Could you check a few things on this model? Use its own coordinates, in mm. Coordinates: 2 decimals unless noted, no trailing zeros. Write each loop counter-clockwise with the first axis right and the second up, starting at its lowest first coordinate (ties: lowest second). Pieces come first, ordered by that corner, then holes. Notation, with made-up numbers: M 25,80.25 L 60,80.25 A26 ccw 60,99.25 Z; hole C -10,22 d2. An arc over 180 degrees is marked long. Answer as CSV lines item,"result". Start each with the question number.
Item 1: I'm going to push flat-ended pins straight in: P1, Ø8, axis at x = -7.5, y = 6.5, coming from the +Z side; P2, Ø3, axis at y = 6, z = 58, coming from the +X side; P3, Ø6, axis at x = -14.5, z = 56.5, coming from the +Y side. Where does each tip first touch, or does it pass through?
Item 2: Suppose I cut it at A-A, the plane z = 27. Write out the boundary of the cut face in (x, y).
Item 3: Suppose I cut it at B-B, the plane y = 15.75. Write out the boundary of the cut face in (x, z).
Item 4: If I drill on line 1 along Y through (x, z) = (-3, 68); line 2 along X through (y, z) = (11.5, 32); line 3 along Y through (x, z) = (-14.75, 41), over which ranges is the centre line in solid material (lowest first)? Write a range as [from, to].
```python
from build123d import *

# Parameters (mm, degrees)
SALIENTE_EXTRUIR1_DEPTH = 77
CORTAR_EXTRUIR1_REACH   = 15.696
CROQUIS2_R              = 1.6


with BuildPart() as part:
    # Croquis1 → Saliente-Extruir1 (new body)
    with BuildSketch(Plane.XY):
        Polygon((-22, 0), (-17.180905327, 0), (0, 13.666629237), (0, 17.5), align=None)
    extrude(amount=SALIENTE_EXTRUIR1_DEPTH)

    # Croquis2 → Cortar-Extruir1 (cut, up to next)
    with BuildSketch(Plane(origin=(-8.52578298, 10.718127175, 0), x_dir=(0.782601054, 0.622523566, 0), z_dir=(-0.622523566, 0.782601054, 0)), mode=Mode.PRIVATE) as cortar_extruir1_sk1:
        with Locations((1.507798766, -5)):
            Circle(CROQUIS2_R)
    cortar_extruir1_tool1 = extrude(cortar_extruir1_sk1.sketch, amount=-CORTAR_EXTRUIR1_REACH, mode=Mode.PRIVATE) & part.part
    add(cortar_extruir1_tool1.solids().sort_by_distance((-7.345778, 11.656767, 5))[0], mode=Mode.SUBTRACT)
    # Croquis2 → Cortar-Extruir1 (cut, up to next)
    with BuildSketch(Plane(origin=(-8.52578298, 10.718127175, 0), x_dir=(0.782601054, 0.622523566, 0), z_dir=(-0.622523566, 0.782601054, 0)), mode=Mode.PRIVATE) as cortar_extruir1_sk2:
        with Locations((1.507798766, -72)):
            Circle(CROQUIS2_R)
    cortar_extruir1_tool2 = extrude(cortar_extruir1_sk2.sketch, amount=-CORTAR_EXTRUIR1_REACH, mode=Mode.PRIVATE) & part.part
    add(cortar_extruir1_tool2.solids().sort_by_distance((-7.345778, 11.656767, 72))[0], mode=Mode.SUBTRACT)


solid = part.part
```
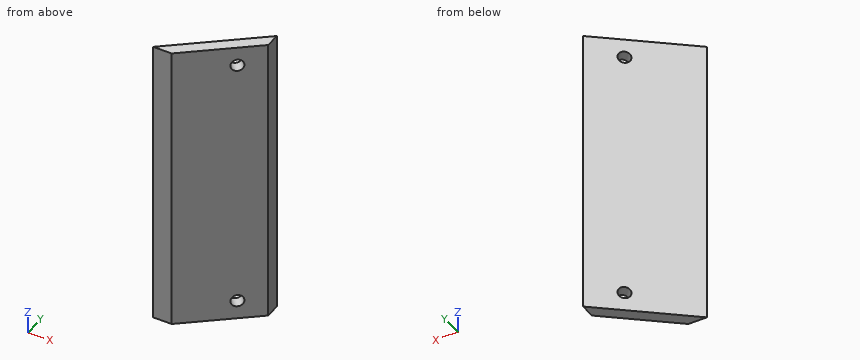
Ans:
1,P1,"stops at z = 77"
1,P2,"stops at x = -7.75"
1,P3,"stops at y = 8.35"
2,outline,"M -22,0 L -17.18,0 L 0,13.67 L 0,17.5 Z"
3,outline,"M -2.2,0 L 0,0 L 0,77 L -2.2,77 Z"
4,line 1,"y = [11.28, 15.11]"
4,line 2,"x = [-7.54, -2.72]"
4,line 3,"y = [1.93, 5.77]"
